Geometry: final body of the model. Coordinates: model frame, mm. Face numbers are marked on the shaded views. A direction names the side the tool comes from. Coordinates: 2 decimals unless noted, no trailing zeros. Loops run counter-clockwise (first coordinate to the right, second up) from the corner with the lowest first, then second, coordinate; pieces in that order, holes last. Notation, with made-up numbers: (-23.75, 47.25) -> (-18.75, 47.25) arc R33 ccw to (-18.75, 80.25) -> close; hole circle Ø8 at (13, 7.5). An arc over 180 degrees is marked (long way). One line per item, written item: value. Start each with the question number.
from build123d import *

# Parameters (mm, degrees)
SKETCH_1_R          = 30
SKETCH_1_R_2        = 27.5
EXTRUDE_1_DEPTH     = 13
SKETCH_1_R_3        = 29.999999999999996
EXTRUDE_1_2_DEPTH   = 13
EXTRUDE_1_3_DEPTH   = 13
EXTRUDE_2_DEPTH     = 2
SKETCH_3_R          = 1.149999999999996
SKETCH_3_R_2        = 1.1499999999999966
SKETCH_3_R_3        = 1.1500000000000037
CUT_EXTRUDE_5_DEPTH = 132.10250765535577
FILLET_1_R          = 10
SKETCH_5_R          = 12.500000000000002
SKETCH_5_R_2        = 10.5
EXTRUDE_3_DEPTH     = 7


with BuildPart() as part:
    # Sketch 1 → Extrude 1 (new body)
    with BuildSketch(Plane.XY):
        with Locations(Location((0, 0, 0), (0, 0, 180))):
            Circle(SKETCH_1_R)
        with Locations(Location((0, 0, 0), (0, 0, 180))):
            Circle(SKETCH_1_R_2, mode=Mode.SUBTRACT)
    extrude(amount=EXTRUDE_1_DEPTH)



with BuildPart() as body_2:
    # Sketch 1 → Extrude 1 2 (new body)
    with BuildSketch(Plane.XY):
        with Locations(Location((66.6, 0, 0), (0, 0, 180))):
            Circle(SKETCH_1_R_3)
        with Locations(Location((66.6, 0, 0), (0, 0, 180))):
            Circle(SKETCH_1_R_2, mode=Mode.SUBTRACT)
    extrude(amount=EXTRUDE_1_2_DEPTH)


with BuildPart() as body_3:
    # Sketch 1 → Extrude 1 3 (new body)
    with BuildSketch(Plane.XY):
        with Locations(Location((33.30000000000001, -57.6772918920436, 0), (0, 0, 180))):
            Circle(SKETCH_1_R_3)
        with Locations(Location((33.30000000000001, -57.6772918920436, 0), (0, 0, 180))):
            Circle(SKETCH_1_R_2, mode=Mode.SUBTRACT)
    extrude(amount=EXTRUDE_1_3_DEPTH)


with BuildPart() as part_1:
    add(part.part)

    add(body_2.part)  # Extrude 2 merges body 2

    add(body_3.part)  # Extrude 2 merges body 3
    # Sketch 2 → Extrude 2 (add)
    with BuildSketch(Plane.XY):
        with BuildLine():
            Line((26.3198925252566, 18.070831312697457), (40.280107474743396, 18.070831312697457))
            ThreePointArc((40.280107474743396, 18.070831312697457), (42.3441853289733, 18.516758123597654), (44.04009212120862, 19.77499826802639))
            ThreePointArc((44.04009212120862, 19.77499826802639), (92.58076211353317, 15), (72.44569692050842, -29.424952464083248))
            ThreePointArc((72.44569692050842, -29.424952464083248), (70.50807559525407, -30.264530756395246), (69.08985272167097, -31.829111208097117))
            Line((69.08985272167097, -31.829111208097117), (62.10974524692759, -43.91901199664395))
            ThreePointArc((62.10974524692759, -43.91901199664395), (61.46389026628078, -45.92951925924603), (61.70560479929982, -48.027337695986766))
            ThreePointArc((61.70560479929982, -48.027337695986766), (33.300000000000004, -87.6772918920436), (4.894395200700185, -48.02733769598677))
            ThreePointArc((4.894395200700185, -48.02733769598677), (5.13610973371921, -45.92951925924604), (4.4902547530724135, -43.91901199664397))
            Line((4.4902547530724135, -43.91901199664397), (-2.489852721670984, -31.829111208097103))
            ThreePointArc((-2.489852721670984, -31.829111208097103), (-3.9080755952540875, -30.264530756395228), (-5.845696920508439, -29.42495246408323))
            ThreePointArc((-5.845696920508439, -29.42495246408323), (-25.980762113533153, 15.000000000000009), (22.55990787879137, 19.77499826802639))
            ThreePointArc((22.55990787879137, 19.77499826802639), (24.25581467102669, 18.516758123597654), (26.3198925252566, 18.070831312697457))
        make_face()
    extrude(amount=EXTRUDE_2_DEPTH)

    # Sketch 3 → Cut-Extrude 5 (cut, through all)
    with BuildSketch(Plane.XY):
        with Locations(Location((33.3, -19.225763964014533, 0), (0, 0, 180))):
            Circle(SKETCH_3_R)
        with Locations(Location((33.3, -12.225763964014533, 0), (0, 0, 180))):
            Circle(SKETCH_3_R_2)
        with Locations(Location((40.3, -19.225763964014533, 0), (0, 0, 180))):
            Circle(SKETCH_3_R)
        with Locations(Location((33.3, -26.22576396401453, 0), (0, 0, 180))):
            Circle(SKETCH_3_R)
        with Locations(Location((26.299999999999997, -19.225763964014533, 0), (0, 0, 180))):
            Circle(SKETCH_3_R_3)
    extrude(amount=CUT_EXTRUDE_5_DEPTH, mode=Mode.SUBTRACT)

    # Fillet 1
    # the kernel refuses this fillet: 10 mm, written as the material it takes off along each edge
    with BuildSketch(Plane(origin=(0, 0, 13), x_dir=(-1, 1.2e-16, 0), z_dir=(1.2e-16, 1, 0))) as fillet_1_piece_1:
        with BuildLine():
            CenterArc((37.5, -6.614378277661482), FILLET_1_R, 138.59037789072914, 41.409622109270856)
            Line((27.5, -6.614378277661482), (27.3, -6.614378277661482))
            Line((27.3, -6.614378277661482), (27.3, 0))
            Line((27.3, 0), (27.5, 0.1999999999999993))
            ThreePointArc((27.5, 0.1999999999999993), (28.75, 0.1999999999999993), (29.85, 0.1322875655532254))
            Line((29.85, 0.1322875655532254), (30, -3.55e-15))
        make_face()
    revolve(axis=Axis((0, 0, 13), (0, 0, 1)), mode=Mode.SUBTRACT)
    with BuildSketch(Plane(origin=(66.6, 0, 13), x_dir=(-1, 1.2e-16, 0), z_dir=(1.2e-16, 1, 0))) as fillet_1_piece_2:
        with BuildLine():
            CenterArc((37.5, -6.614378277661482), FILLET_1_R, 138.59037789072914, 41.409622109270856)
            Line((27.5, -6.614378277661482), (27.299999999999997, -6.614378277661482))
            Line((27.299999999999997, -6.614378277661482), (27.299999999999997, 0))
            Line((27.299999999999997, 0), (27.5, 0.1999999999999993))
            ThreePointArc((27.5, 0.1999999999999993), (28.75, 0.1999999999999993), (29.85, 0.1322875655532254))
            Line((29.85, 0.1322875655532254), (30, -3.55e-15))
        make_face()
    revolve(axis=Axis((66.6, 0, 13), (0, 0, 1)), mode=Mode.SUBTRACT)
    with BuildSketch(Plane(origin=(33.30000000000001, -57.6772918920436, 13), x_dir=(-1, 0, 0), z_dir=(0, 1, 0))) as fillet_1_piece_3:
        with BuildLine():
            CenterArc((37.5, -6.614378277661478), FILLET_1_R, 138.59037789072914, 41.409622109270856)
            Line((27.5, -6.614378277661478), (27.3, -6.614378277661478))
            Line((27.3, -6.614378277661478), (27.3, 0))
            Line((27.3, 0), (27.5, 0.1999999999999993))
            ThreePointArc((27.5, 0.1999999999999993), (28.75, 0.1999999999999993), (29.849999999999998, 0.1322875655532254))
            Line((29.849999999999998, 0.1322875655532254), (30, -3.55e-15))
        make_face()
    revolve(axis=Axis((33.30000000000001, -57.6772918920436, 13), (0, 0, 1)), mode=Mode.SUBTRACT)

    # Sketch 5 → Extrude 3 (add)
    with BuildSketch(Plane(origin=(0, 0, 0), x_dir=(-1, 0, 0), z_dir=(0, 0, -1))):
        with Locations(Location((-33.3, -19.225763964014533, 0), (0, 0, 180))):
            Circle(SKETCH_5_R)
        with Locations((-33.3, -19.225763964014533)):
            Circle(SKETCH_5_R_2, mode=Mode.SUBTRACT)
    extrude(amount=EXTRUDE_3_DEPTH)


solid = part_1.part
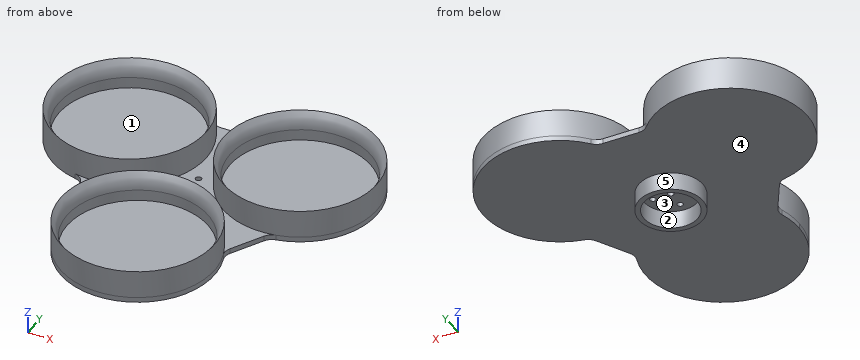
1. Set-up query: the marked faces 1 and 2. Return all of +Z, -Z, +X, -X, +Y, -Y with unobstructed straight access to the full face (end or side cutting, diameter ignored); none if empty.
2. Pin query (flat end, axial travel): pin 1 Ø4 at (y, z) = (-73, 2.5) entering from -X; pin 2 Ø12 at (x, z) = (68, 2) entering from +Y; pin 3 Ø4 at (y, z) = (-35, 7) entering from +X; pin 4 Ø1.4 at (x, y) = (40.3, -19.23) entering from -Z. Return the tip coordinate at first contact, or that it passes through.
3. Draft query along X for the marked faces 3, 4 and 5. Return one class per face: released by +X, released by -X, zero draft, split by the parting line, or undercut.
4. Line query: L1, parallel to Y at x = 33.3, z = 5.2; L2, parallel to Z at x = -6, y = 10; L3, parallel to Y at x = 66.5, z = 9.5. Output: solid intervals per line, ascending. Write a range as [from, to].
5. Section B-B on z = -4. Return the cut outline in (x, y).
6. Section A-A on x = 66.6. Return the cut outline in (y, z), plus the area to 3 significant figures.
Checks:
1. face 1: +Z
1. face 2: -Z
2. pin 1: x = 6.42
2. pin 2: y = 30
2. pin 3: x = 55.04
2. pin 4: through
3. face 3: undercut
3. face 4: zero draft
3. face 5: split by the parting line
4. L1: [-87.68, -85.18], [-30.18, -27.68]
4. L2: [0, 2]
4. L3: [-30, -28], [28, 30]
5. outline: circle Ø25 at (33.3, -19.23); hole circle Ø21 at (33.3, -19.23)
6. outline: (-36.14, 0) -> (30, 0) -> (30, 13) arc R10 ccw to (27.5, 6.39) -> (27.5, 2) -> (-27.5, 2) -> (-27.5, 6.39) arc R10 ccw to (-30, 13) -> (-30, 2) -> (-36.14, 2) -> close
6. area: 177 mm²
